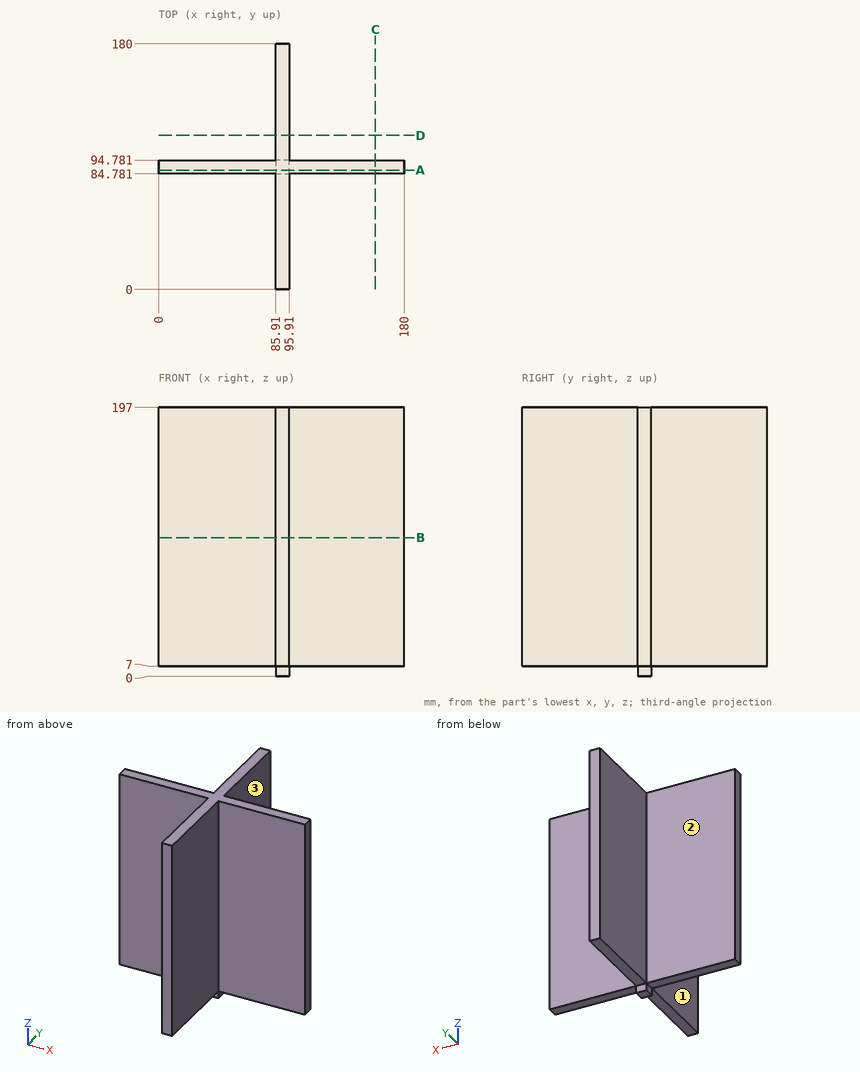
Design review of the part shown in the three views and the two pictorial views. Dimensions are in mm from the part's minimum x, y and z. A direction names the side the tool comes from. Coordinates: 2 decimals unless noted, no trailing zeros. Write each loop counter-clockwise with the first axis right and the second up, starting at its lowest first coordinate (ties: lowest second). Pieces come first, ordered by that corner, then holes.
1) To check wall thickness, follow probe 1 along X at (y, z) = (32, 99); probe 2 along Z at (x, y) = (88.5, 129); probe 3 along Y at (x, z) = (140, 140). State the ranges of each line that lie inside material, in increasing order.
2) Clearance check with flat-ended pins moving along their axes: pin 1 Ø2 at (y, z) = (115, 142.5) entering from -X; pin 2 Ø1 at (x, z) = (61, 82) entering from -Y; pin 3 Ø5 at (x, y) = (121.5, 89.5) entering from -Z. State where each tip first meets the part, or that it passes through.
3) We need section C-C on x = 159. State the section outline as (y, z) points.
4) We need section D-D on y = 113. State the section outline as (x, z) points, then the cut area to 3 significant figures.
5) We need section B-B on z = 101.5. State the section outline as (x, y) points, then the cut area to 3 significant figures.
6) We need section A-A on y = 87.5. State the section outline as (x, z) points, then the cut area to 3 significant figures.
7) Machinability: for the marked faces 1, 2 and 3, which of the approach directions +Z, -Z, +X, -X, +Y, -Y give a long, thin tool a straight path to every point of the face, cutting with its end or side? Answer none if there is none.
Answer list:
1. probe 1: x = 85.91 to 95.91
1. probe 2: z = 7 to 197
1. probe 3: y = 84.78 to 94.78
2. pin 1: stops at x = 85.91
2. pin 2: stops at y = 84.78
2. pin 3: stops at z = 7
3. outline: (84.78, 7) - (94.78, 7) - (94.78, 197) - (84.78, 197) - close
4. outline: (85.91, 7) - (95.91, 7) - (95.91, 197) - (85.91, 197) - close
4. area: 1,900 mm2
5. outline: (0, 84.78) - (85.91, 84.78) - (85.91, 0) - (95.91, 0) - (95.91, 84.78) - (180, 84.78) - (180, 94.78) - (95.91, 94.78) - (95.91, 180) - (85.91, 180) - (85.91, 94.78) - (0, 94.78) - close
5. area: 3,500 mm2
6. outline: (0, 7) - (85.91, 7) - (85.91, 0) - (95.91, 0) - (95.91, 7) - (180, 7) - (180, 197) - (0, 197) - close
6. area: 34,300 mm2
7. face 1: +Z, -Z, -X, -Y
7. face 2: +Z, -Z, -X, +Y
7. face 3: +Z, -Z, +X, +Y
